from build123d import *

# Parameters (mm, degrees)
F0_R     = 5
F1_DEPTH = 12.7


with BuildPart() as f1:
    # F0 (on Front) → F1 (new body, symmetric)
    with BuildSketch(Plane.XZ):
        with BuildLine():
            ThreePointArc((-49, 9.949874), (-60, 0), (-49, -9.949874))
            ThreePointArc((-49, -9.949874), (-43.30127, -25), (-33.116844, -37.460308))
            ThreePointArc((-33.116844, -37.460308), (-30, -51.961524), (-15.883156, -47.410182))
            ThreePointArc((-15.883156, -47.410182), (0, -50), (15.883156, -47.410182))
            ThreePointArc((15.883156, -47.410182), (30, -51.961524), (33.116844, -37.460308))
            ThreePointArc((33.116844, -37.460308), (43.30127, -25), (49, -9.949874))
            ThreePointArc((49, -9.949874), (60, 0), (49, 9.949874))
            ThreePointArc((49, 9.949874), (43.30127, 25), (33.116844, 37.460308))
            ThreePointArc((33.116844, 37.460308), (30, 51.961524), (15.883156, 47.410182))
            ThreePointArc((15.883156, 47.410182), (0, 50), (-15.883156, 47.410182))
            ThreePointArc((-15.883156, 47.410182), (-30, 51.961524), (-33.116844, 37.460308))
            ThreePointArc((-33.116844, 37.460308), (-43.30127, 25), (-49, 9.949874))
        make_face()
        with Locations((-25, -43.30127)):
            Circle(F0_R, mode=Mode.SUBTRACT)
        with Locations((25, -43.30127)):
            Circle(F0_R, mode=Mode.SUBTRACT)
        with BuildLine():
            ThreePointArc((28.284271, -28.284271), (15.307337, -36.955181), (0, -40))
            ThreePointArc((0, -40), (-5, -35), (0, -30))
            ThreePointArc((0, -30), (11.480503, -27.716386), (21.213203, -21.213203))
            ThreePointArc((21.213203, -21.213203), (28.284271, -21.213203), (28.284271, -28.284271))
        make_face(mode=Mode.SUBTRACT)
        with Locations((-50, 0)):
            Circle(F0_R, mode=Mode.SUBTRACT)
        with BuildLine():
            ThreePointArc((-38.637033, -10.352762), (-39.657794, 5.221048), (-34.641016, 20))
            ThreePointArc((-34.641016, 20), (-27.810889, 21.830127), (-25.980762, 15))
            ThreePointArc((-25.980762, 15), (-29.743346, 3.915786), (-28.977775, -7.764571))
            ThreePointArc((-28.977775, -7.764571), (-32.513309, -13.888296), (-38.637033, -10.352762))
        make_face(mode=Mode.SUBTRACT)
        with Locations((-25, 43.30127)):
            Circle(F0_R, mode=Mode.SUBTRACT)
        with BuildLine():
            ThreePointArc((7.764571, 28.977775), (4.229037, 35.101499), (10.352762, 38.637033))
            ThreePointArc((10.352762, 38.637033), (24.350457, 31.734134), (34.641016, 20))
            ThreePointArc((34.641016, 20), (32.810889, 13.169873), (25.980762, 15))
            ThreePointArc((25.980762, 15), (18.262843, 23.8006), (7.764571, 28.977775))
        make_face(mode=Mode.SUBTRACT)
        with Locations((50, 0)):
            Circle(F0_R, mode=Mode.SUBTRACT)
        with Locations((25, 43.30127)):
            Circle(F0_R, mode=Mode.SUBTRACT)
    extrude(amount=F1_DEPTH, both=True)


solid = f1.part
Model file for the job. Use its own axes, mm. A direction names the side the tool comes from. Give positions to 0.01 mm unless a question says otherwise; leave off trailing zeros. Write each loop counter-clockwise with the first axis right and the second up, starting at its lowest first coordinate (ties: lowest second). Pieces come first, ordered by that corner, then holes. Notation, with made-up numbers: M 32.5,36 L 69.5,36 A17 cw 69.5,42 Z; hole C -20,56.5 d4. An arc over 180 degrees is marked long. One line per item, written item: value. Start each with the question number.
Q1. Drop flat-ended pins along their axis: pin 1 Ø16 at (x, z) = (-25, -43.3) entering from +Y; pin 2 Ø4 at (y, z) = (3.5, 38) entering from +X; pin 3 Ø8 at (x, z) = (25, -43.3) entering from +Y; pin 4 Ø12 at (y, z) = (-7, 12.5) entering from +X. Give the stop position or say it passes through.
Q2. Two-plate mould, pull along X, no slides. Class faces 1 (the flat face through (-1, 12.7, 1)), 2 (the cylindrical face through (20.005, 0.178, -43.081)), 3 (the cylindrical face through (29.796, -0.178, -52.076)): +X half, -X half, draft (parallel to the pull), parting line (faces both ways), or undercut.
Q3. Probe probe 1 along Z at (x, y) = (-25, -4.5); probe 2 along Z at (x, y) = (9, 1); probe 3 along X at (y, z) = (8.75, 20). List the from-to ranges inside material, lowest first. Write a range as [from, to].
Q4. Saw through at D-D, the plane y = -6. State how many separate pieces and enclosed holes the cut face has, plus the area to 3 significant figures.
Q5. Saw through at A-A, the plane z = 0. Write the cut outline in (x, y), plus the area to 3 significant figures.
Q6. Saw through at B-B, the plane x = 1.5. Write the cut outline in (y, z).
Q7. 3-axis set-ups, long thin cutter, end or side, ignore diameter. For faces 4 (the cylindrical face through (-29.72, -0.18, 4.08)), 5 (the cylindrical face through (0, 0, -50)): which of +Z, -Z, +X, -X, +Y, -Y reach the whole face in a straight line?
Q8. Saw through at C-C, the plane z = -35. Write the cut outline in (x, y).
Output values:
1. pin 1: stops at y = 12.7
1. pin 2: stops at x = 34.7
1. pin 3: passes through
1. pin 4: stops at x = 57.6
2. face 1: draft
2. face 2: undercut
2. face 3: undercut
3. probe 1: z = [-53.3, -48.3], [-38.3, 38.3], [48.3, 53.3]
3. probe 2: z = [-49.18, -38.97], [-28.62, 28.62], [38.81, 49.18]
3. probe 3: x = [-45.83, -34.64], [-25.98, 22.36], [34.64, 45.83]
4. separate pieces: 1
4. enclosed holes: 9
4. area: 7,300 mm²
5. outline: M -60,-12.7 L -55,-12.7 L -55,12.7 L -60,12.7 Z; M -45,-12.7 L -40,-12.7 L -40,12.7 L -45,12.7 Z; M -30,-12.7 L 45,-12.7 L 45,12.7 L -30,12.7 Z; M 55,-12.7 L 60,-12.7 L 60,12.7 L 55,12.7 Z
5. area: 2,290 mm²
6. outline: M -12.7,-49.98 L 12.7,-49.98 L 12.7,-39.97 L -12.7,-39.97 Z; M -12.7,-29.96 L 12.7,-29.96 L 12.7,49.98 L -12.7,49.98 Z
7. face 4: +Y, -Y
7. face 5: -Z, +Y, -Y
8. outline: M -35.71,-12.7 L -5,-12.7 L -5,12.7 L -35.71,12.7 Z; M 19.36,-12.7 L 35.71,-12.7 L 35.71,12.7 L 19.36,12.7 Z
